```python
from build123d import *

# Parameters (mm, degrees)
SKETCH_1_W          = 174.091607372
SKETCH_1_H          = 60.823122747
EXTRUDE_1_DEPTH     = 2
SKETCH_2_R          = 6.75
SKETCH_2_R_2        = 4
SKETCH_2_R_3        = 6.387609309
CUT_EXTRUDE_2_DEPTH = 3
SKETCH_5_R          = 2.8
SKETCH_5_R_2        = 3.2
CUT_EXTRUDE_6_DEPTH = 3


with BuildPart() as part:
    # Эскиз1 → Бобышка-Вытянуть1 (new body)
    with BuildSketch(Plane.XY):
        with Locations((41.416369032, 15.037436288)):
            Rectangle(SKETCH_1_W, SKETCH_1_H)
    extrude(amount=EXTRUDE_1_DEPTH)

    # Эскиз2 → Вырез-Вытянуть2 (cut, through all)
    with BuildSketch(Plane.XY.offset(2)):
        with Locations((-19.785334363, 17.425924278)):
            Circle(SKETCH_2_R)
        with Locations((26.791510955, 5.539037957)):
            Circle(SKETCH_2_R_2)
        with Locations((35.178515275, 5.052050609)):
            Circle(SKETCH_2_R_2)
        with Locations((105.297300125, 18.321325083)):
            Circle(SKETCH_2_R_3)
    extrude(amount=-CUT_EXTRUDE_2_DEPTH, mode=Mode.SUBTRACT)

    # Эскиз5 → Вырез-Вытянуть6 (cut, through all)
    with BuildSketch(Plane.XY.offset(2)):
        with Locations((91.162128274, 26.645923824)):
            Circle(SKETCH_5_R)
        with Locations((91.162128274, 9.6)):
            Circle(SKETCH_5_R)
        with Locations((42.296935023, 5.602595819)):
            Circle(SKETCH_5_R_2)
        Polygon((28.570706192, 9.34764981), (28.570706192, -16.12332621), (32.666265218, -16.12332621), (32.666265218, 9.330532976), align=None)
        Polygon((33.503712587, 38.765606149), (19.738187242, 20.818838125), (17.024936958, 23.734062815), (-4.96394501, 51.572688279), (27.970840429, 51.572688279), align=None)
        Polygon((31.662167761, 46.983470514), (39.910203219, 24.587362026), (58.988646835, 46.983470514), align=None)
        Polygon((4.611696012, -1.281488831), (17.024936958, -1.281488831), (19.738187242, -15.374125086), (1.915533217, -15.374125086), align=None)
        Polygon((-5.563318521, -15.374125086), (-3.57038705, 8.280770389), (-3.57038705, 19.874672628), (-5.563318521, 50.475189584), (-48.013678964, 50.475189584), (-48.013678964, -15.374125086), align=None)
        Polygon((72.33728383, 15.460155755), (65.492559947, 3.970797808), (45.936205994, 3.970797808), (41.416369032, -15.374125086), (128.462172718, -15.374125086), (128.462172718, 45.448997661), (111.938900584, 3.970797808), (79.915370987, 3.970797808), align=None)
        Polygon((61.092380308, 47.449740359), (52.544642812, 37.635973837), (105.888722073, 35.749872981), (103.242302386, 29.670868316), (110.190804078, 26.645923824), (113.207690043, 32.789853089), (118.919189497, 23.734062815), (126.889373288, 45.448997661), align=None)
    extrude(amount=-CUT_EXTRUDE_6_DEPTH, mode=Mode.SUBTRACT)


solid = part.part
```
CAD build for the part. Positions are in the model's coordinates, mm. A direction names the side the tool comes from. Round coordinates to 2 decimals unless told otherwise and drop trailing zeros. Write each loop counter-clockwise with the first axis right and the second up, starting at its lowest first coordinate (ties: lowest second). Pieces come first, ordered by that corner, then holes.
Item 1: Drop flat-ended pins along their axis: pin 1 Ø1.5 at (x, y) = (102.5, 11.5) entering from -Z; pin 2 Ø1 at (x, z) = (13, 0.5) entering from -Y; pin 3 Ø0.6 at (y, z) = (-7, 1.5) entering from +X; pin 4 Ø0.6 at (y, z) = (-4.5, 0.5) entering from -X. Give the stop position or say it passes through.
Filled in:
pin 1: stops at z = 0
pin 2: stops at y = -1.28
pin 3: stops at x = 43.44
pin 4: stops at x = -4.67
Item 2: Mould opens along Y. For faces 5 (the cylindrical face through (22.793, 5.653, 1.014)), 6 (the flat face through (106.67, 28.18, 1.01)), 7 (the flat face through (68.963, 9.796, 1.014)), 8 (the flat face through (18.401, 22.256, 1.014)) say: released by +Y, released by -Y, zero draft, split by the parting line, or undercut.
Filled in:
face 5: undercut
face 6: undercut
face 7: released by -Y
face 8: released by +Y
Item 3: Drill centre lines: L1, parallel to X at y = 14.5, z = 1.35; L2, parallel to Y at x = 105, z = 0.45; L3, parallel to X at y = 35, z = 0.65. Where is each one in solid material? Low to high.
Filled in:
L1: x = -3.57 to 71.77, 72.97 to 100.18, 110.42 to 116.13
L2: y = 3.97 to 11.94, 24.7 to 28.91, 33.71 to 35.78
L3: x = -4.56 to 8.13, 30.62 to 36.08, 48.78 to 105.56, 123.05 to 124.3
Item 4: Band-saw the part on A-A on y = 42.5. Write the cut outline in (x, z).
Filled in:
outline: (-5.04, 0) - (2.2, 0) - (2.2, 2) - (-5.04, 2) - close; (31.89, 0) - (33.31, 0) - (33.31, 2) - (31.89, 2) - close; (55.17, 0) - (56.78, 0) - (56.78, 2) - (55.17, 2) - close; (125.81, 0) - (127.29, 0) - (127.29, 2) - (125.81, 2) - close
Item 5: Band-saw the part on B-B on z = 1.45. Give the number of separate pieces and of enclosed holes in the cut face, then the cut area to 3 significant figures.
Filled in:
separate pieces: 1
enclosed holes: 3
area: 3,920 mm2
Item 6: Tool access for faces 1 (the flat face through (18.363, -8.229, 1.014)), 2 (the flat face through (104.584, 32.753, 1.014)), 3 (the flat face through (43.7, -5.6, 1)), 4 (the flat face through (122.85, 34.44, 1.01)): list every direction of +Z, -Z, +X, -X, +Y, -Y with a clear straight run to the whole face (end or side of a thin tool).
Filled in:
face 1: +Z, -Z, -Y
face 2: +Z, -Z
face 3: +Z, -Z, +X, -Y
face 4: +Z, -Z, +Y
